Autodesk Inventor part; units mm, degrees
ref_plane "YZ Plane" through (0, 0, 0) normal (1, 0, 0) x (0, 1, 0)
ref_plane "XZ Plane" through (0, 0, 0) normal (0, 1, 0) x (-1, 0, 0)
ref_plane "XY Plane" through (0, 0, 0) normal (0, 0, 1) x (1, 0, 0)
sketch "Sketch1" plane through (0, 0, 0) normal (0, 0, 1) x (1, 0, 0)
  circle A0 centre (0, 0) radius 16
  dimension "d0" = 32
extrude "Extrusion1" add sketch "Sketch1" along normal blind 7.8
sketch "Sketch2" plane through (0, 0, 7.8) normal (0, 0, 1) x (1, 0, 0)
  circle A0 centre (0, 0) radius 16
  circle A1 centre (0, 0) radius 6
  dimension "d3" = 12
extrude "Extrusion2" add sketch "Sketch2" along normal blind 46 contours A1
sketch "Sketch3" plane through (0, 0, 53.8) normal (0, 0, 1) x (1, 0, 0)
  circle A0 centre (0, 0) radius 6
  circle A1 centre (0, 0) radius 2.75
  dimension "d6" = 5.5
extrude "Extrusion3" cut sketch "Sketch3" against normal blind 15 contours A1
chamfer "Chamfer1" distance 1 angle 45 1 edges at (-6, 0, 53.8)
properties part number "piston" material "Stainless Steel"
Source: CAD feature listing. Evaluate the final solid. Frame: model axes, mm. A direction names the side the tool comes from. Give positions to 0.01 mm unless a question says otherwise; leave off trailing zeros. Write each loop counter-clockwise with the first axis right and the second up, starting at its lowest first coordinate (ties: lowest second). Pieces come first, ordered by that corner, then holes. Notation, with made-up numbers: (80, -5) - (107, -5) arc R33 cw to (107, 27) - close; hole circle Ø2 at (-26.5, 6.25). An arc over 180 degrees is marked (long way). One line per item, written item: value. Start each with the question number.
Q1. Material intervals for probe 1 along Y at (x, z) = (0, 44); probe 2 along Z at (x, y) = (-1.5, -15); probe 3 along Y at (x, z) = (5, 49), sorted ascending. Write a range as from..to.
Q2. Section query D-D, the plane z = 23. Return the cut outline in (x, y), then the cut area to 3 significant figures.
Q3. Section query A-A, the plane x = 0. Return the cut outline in (y, z).
Q4. Section query C-C, the plane z = 43.5. Return the cut outline in (x, y).
Q5. Draft query along Y for faces 3 (the face through (0, 0, 38.8)), 4 (the face through (-3.47, 15.62, 3.85)), 5 (the face through (7, 0, 7.8)), 6 (the face through (-0.596, -2.685, 46.405)). Return one class per face: +Y half, -Y half, draft (parallel to the pull), parting line (faces both ways), or undercut.
Q6. Set-up query: faces 1 (the face through (-6, 0, 30)), 2 (the face through (2.2, -2.2, 53.8)). Return all of +Z, -Z, +X, -X, +Y, -Y with unobstructed straight access to the full face (end or side cutting, diameter ignored); none if empty.
Q7. First-contact query: pin 1 Ø8 at (y, z) = (8.5, 12) entering from -X; pin 2 Ø10 at (y, z) = (2, 16.5) entering from +X; pin 3 Ø12 at (x, z) = (-2.5, 43.5) entering from -Y. Flat tips, straight axial feed; report the tip coordinate or a pass-through.
Answer:
1. probe 1: y = -6..-2.75, 2.75..6
1. probe 2: z = 0..7.8
1. probe 3: y = -3.32..3.32
2. outline: circle Ø12 at (0, 0)
2. area: 113 mm2
3. outline: (-16, 0) - (16, 0) - (16, 7.8) - (6, 7.8) - (6, 52.8) - (5, 53.8) - (2.75, 53.8) - (2.75, 38.8) - (-2.75, 38.8) - (-2.75, 53.8) - (-5, 53.8) - (-6, 52.8) - (-6, 7.8) - (-16, 7.8) - close
4. outline: circle Ø12 at (0, 0); hole circle Ø5.5 at (0, 0)
5. face 3: undercut
5. face 4: parting line
5. face 5: draft
5. face 6: undercut
6. face 1: +Z
6. face 2: +Z, +X, -X, +Y, -Y
7. pin 1: stops at x = -3.97
7. pin 2: stops at x = 6
7. pin 3: stops at y = -6
